Here's how the part is built. I have some questions about the finished solid (model axes, mm). Face numbers are marked on the shaded views. Give positions to 0.01 mm unless a question says otherwise; leave off trailing zeros. Order: outer loops, then holes, each group sorted by start corner. A loop starts at its lowest first (then second) coordinate and runs counter-clockwise, first axis right, second up.
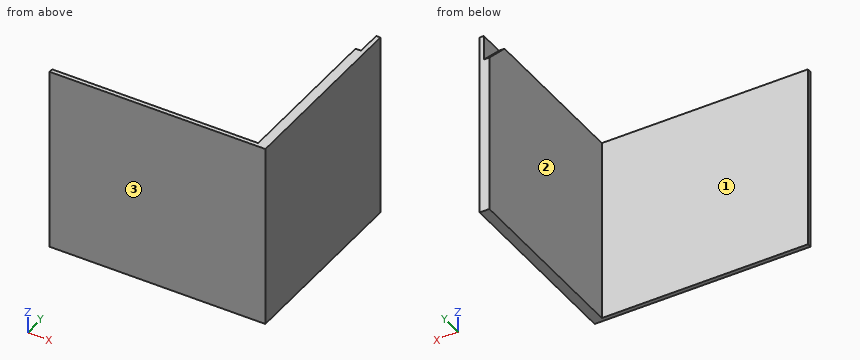
Autodesk Inventor part; units mm, degrees
ref_plane "YZ Plane" through (0, 0, 0) normal (1, 0, 0) x (0, 1, 0)
ref_plane "XZ Plane" through (0, 0, 0) normal (0, 1, 0) x (-1, 0, 0)
ref_plane "XY Plane" through (0, 0, 0) normal (0, 0, 1) x (1, 0, 0)
sketch "Sketch1" plane through (0, 0, 0) normal (0, 1, 0) x (-1, 0, 0)
  line L0 (110, -80) -> (-110, -80)
  line L1 (-110, -80) -> (-110, 80)
  line L2 (-110, 80) -> (110, 80)
  line L3 (110, 80) -> (110, -80)
  line L4 (320.2117, -53.5522) -> (168.036, -53.5522) construction
  line L5 (168.036, -53.5522) -> (168.036, 90.1689) construction
  line L6 (168.036, 90.1689) -> (320.2117, 90.1689) construction
  line L7 (320.2117, 90.1689) -> (320.2117, -53.5522) construction
  line L8 (124.3, -89.75) -> (-124.3, -89.75) construction
  line L9 (-124.3, -89.75) -> (-124.3, 89.75) construction
  line L10 (-124.3, 89.75) -> (124.3, 89.75) construction
  line L11 (124.3, 89.75) -> (124.3, -89.75) construction
  line L12 (124.3, -89.75) -> (-124.3, 89.75) construction
  line L13 (-124.3, -89.75) -> (124.3, 89.75) construction
  line L14 (-152.4, -107.95) -> (152.4, -107.95)
  line L15 (152.4, -107.95) -> (152.4, 107.95)
  line L16 (152.4, 107.95) -> (-152.4, 107.95)
  line L17 (-152.4, 107.95) -> (-152.4, -107.95)
  line L18 (-152.4, -107.95) -> (152.4, 107.95) construction
  line L19 (152.4, -107.95) -> (-152.4, 107.95) construction
  line L20 (177.8, 133.35) -> (177.8, -133.35)
  line L21 (177.8, -133.35) -> (-177.8, -133.35)
  line L22 (-177.8, -133.35) -> (-177.8, 133.35)
  line L23 (-177.8, 133.35) -> (177.8, 133.35)
  point P0 (0, 0)
  dimension "d11" = 220
  dimension "d12" = 160
  dimension "d15" = 248.6
  dimension "d16" = 179.5
  dimension "d18" = 304.8
  dimension "d19" = 215.9
  dimension "d22" = 25.4
extrude "Top" add sketch "Sketch1" along normal blind 25.4 contours L17 L16 L15 L14 | L20 L21 L22 L23
sketch "Sketch3" plane through (177.8, 0, 133.35) normal (1, 0, 0) x (0, 0, -1)
  line L0 (0, 0) -> (0, 25.4)
  line L1 (266.7, 0) -> (266.7, 25.4)
  line L2 (0, 0) -> (266.7, 0)
  line L3 (266.7, 0) -> (266.7, -266.7)
  line L4 (266.7, -266.7) -> (0, -266.7)
  line L5 (0, -266.7) -> (0, 0)
  point P0 (133.35, 0)
  dimension "d25" = 266.7
extrude "Right" add sketch "Sketch3" against normal blind 50.8
sketch "Sketch4" plane through (-177.8, 0, -133.35) normal (-1, 0, 0) x (0, 0, 1)
  line L0 (0, 0) -> (0, 25.4)
  line L1 (266.7, -266.7) -> (266.7, 0)
  line L2 (0, 0) -> (266.7, 0)
  line L3 (266.7, 0) -> (266.7, -266.7)
  line L4 (266.7, -266.7) -> (0, -266.7)
  line L5 (0, -266.7) -> (0, 0)
  point P0 (133.35, 0)
  dimension "d28" = 266.7
extrude "Left" add sketch "Sketch4" against normal blind 50.8
sketch "Sketch5" plane through (0, 0, 0) normal (1, 0, 0) x (0, 1, 0)
  line L0 (-266.7, -133.35) -> (25.4, -133.35)
  line L1 (-266.7, 133.35) -> (-266.7, -133.35)
  line L2 (0, -133.35) -> (-266.7, 133.35)
  line L3 (-266.7, 133.35) -> (-275.6803, 124.3697)
  line L4 (-275.6803, 124.3697) -> (-8.9803, -142.3303)
  line L5 (-8.9803, -142.3303) -> (0, -133.35)
  point P0 (0, 0)
  dimension "d31" = 12.7
extrude "Plexiglass Cut" cut sketch "Sketch5" along normal mid plane 304.8 contours L4 L1 L2 L0 | L0 L5 L4 | L4 L3 L1
sketch "Sketch6" plane through (-177.8, -266.7, -133.35) normal (0, -1, 0) x (1, 0, 0)
  line L0 (0, 0) -> (0, 266.7)
  line L1 (355.6, 0) -> (0, 0)
  line L2 (0, 266.7) -> (355.6, 266.7)
  line L3 (355.6, 266.7) -> (355.6, 0)
  line L4 (355.6, 0) -> (0, 0)
  line L5 (0, 0) -> (0, 266.7)
  point P0 (177.8, 133.35)
extrude "Bottom" add sketch "Sketch6" along normal blind 25.4
sketch "Sketch9" plane through (0, 25.4, 0) normal (0, 1, 0) x (1, 0, 0)
  line L0 (177.8, -133.35) -> (127, -133.35)
  line L1 (177.8, 133.35) -> (-177.8, 133.35)
  line L2 (177.8, -133.35) -> (-177.8, -133.35)
  line L3 (-177.8, -133.35) -> (-177.8, 133.35)
  line L4 (-177.8, 133.35) -> (177.8, 133.35)
  line L5 (177.8, 133.35) -> (177.8, -133.35)
  point P0 (0, 0)
extrude "Top Flattening" cut sketch "Sketch9" against normal blind 22.4
sketch "Sketch10" plane through (0, 3, 0) normal (0, 1, 0) x (1, 0, 0)
  line L0 (-177.8, -133.35) -> (-177.8, 133.35)
  line L1 (-155.4106, 133.35) -> (-177.8, 133.35)
  line L2 (-177.8, 133.35) -> (-177.8, -133.35)
  line L3 (-177.8, -133.35) -> (-155.4106, -133.35)
  line L4 (-155.4106, -133.35) -> (-155.4106, 133.35)
  line L5 (177.8, 133.35) -> (177.8, -133.35)
  line L6 (177.8, -133.35) -> (155.4106, -133.35)
  line L7 (155.4106, -133.35) -> (155.4106, 133.35)
  line L8 (155.4106, 133.35) -> (177.8, 133.35)
  line L9 (152.4, -115.3895) -> (152.4, 133.35)
  point P0 (0, 0)
  point P1 (-177.8, 0)
  dimension "d48" = 22.3894
  dimension "d49" = 22.3894
extrude "Outer Side Flattening" cut sketch "Sketch10" against normal through all
sketch "Sketch11" plane through (-177.8, -292.1, -133.35) normal (0, -1, 0) x (1, 0, 0)
  line L0 (22.3894, 0) -> (333.2106, 0)
  line L1 (333.2106, 0) -> (22.3894, 0)
  line L2 (22.3894, 0) -> (22.3894, 266.7)
  line L3 (22.3894, 266.7) -> (333.2106, 266.7)
  line L4 (333.2106, 266.7) -> (333.2106, 0)
  point P0 (177.8, 133.35)
extrude "Bottom Flattening" cut sketch "Sketch11" against normal blind 22.4
sketch "Sketch12" plane through (155.4106, 3, -133.35) normal (0, 0, -1) x (-1, 0, 0)
  line L0 (155.4106, -3) -> (155.4106, -269.7) construction
  line L1 (7.0106, -269.7) -> (7.0106, -3)
  line L2 (7.0106, -3) -> (303.8106, -3)
  line L3 (303.8106, -3) -> (303.8106, -269.7)
  line L4 (303.8106, -269.7) -> (7.0106, -269.7)
  line L5 (7.0106, -269.7) -> (303.8106, -3) construction
  line L6 (7.0106, -3) -> (303.8106, -269.7) construction
  point P0 (155.4106, -136.35)
  point P1 (155.4106, -3)
  dimension "d54" = 296.8
extrude "Inner Flattening" cut sketch "Sketch12" against normal through all
sketch "Sketch13" plane through (-155.4106, 3, 133.35) normal (0, 0, 1) x (1, 0, 0)
  line L0 (310.8211, -272.7) -> (310.8211, 0)
  line L1 (0, -272.7) -> (0, 0)
  line L2 (310.8211, -136.35) -> (0, -136.35)
  line L3 (0, -136.35) -> (0, 0)
  line L4 (0, 0) -> (310.8211, 0)
  line L5 (310.8211, 0) -> (310.8211, -136.35)
  point P0 (155.4106, -3)
  point P1 (310.8211, 0)
  point P2 (0, -136.35)
extrude "Top Cut" cut sketch "Sketch13" against normal through all
sketch "Sketch14" plane through (-155.4106, -133.35, 133.35) normal (0, 1, 0) x (1, 0, 0)
  line L0 (310.8211, 266.7) -> (0, 266.7)
  line L1 (155.4106, 133.35) -> (310.8211, 133.35)
  line L2 (310.8211, 133.35) -> (310.8211, 266.7)
  line L3 (310.8211, 266.7) -> (155.4106, 266.7)
  line L4 (155.4106, 266.7) -> (155.4106, 133.35)
  line L5 (0, 0) -> (310.8212, 0)
  line L6 (310.8211, 266.7) -> (0, 266.7)
  line L7 (0, 266.7) -> (0, 0)
  line L8 (0, 0) -> (310.8211, 0)
  line L9 (310.8211, 0) -> (310.8211, 266.7)
extrude "Quarter Cut" cut sketch "Sketch14" against normal through all contours L4 L1 L9 L5 L7 L0
properties part number "Apple iPad 2022 Hologram"
Q1. If we section it at A-A on z = -96: List the corners of the cut face in (x, y) for me, plus the area to 3 significant figures.
Filled sheet:
outline: (0, -269.7) - (155.41, -269.7) - (155.41, -133.35) - (148.4, -133.35) - (148.4, -266.7) - (0, -266.7) - close
area: 1,400 mm2
Q2. I need wall thicknesses on L1, parallel to X at y = -162, z = -77; L2, parallel to Y at x = 95, z = -104.5. Which ranges of each line are inside material? Lowest first, please.
Filled sheet:
L1: x = 148.4 to 155.41
L2: y = -269.7 to -266.7
Q3. If we section it at C-C on y = -229.5: List the corners of the cut face in (x, z) for me.
Filled sheet:
outline: (148.4, -133.35) - (155.41, -133.35) - (155.41, 0) - (148.4, 0) - close
Q4. Thinking about a two-plate mould opening in Y: for the marked faces 1, 2 and 3, which applies, released by +Y, released by -Y, zero draft, split by the parting line, or undercut?
Filled sheet:
face 1: released by +Y
face 2: zero draft
face 3: released by -Y
Q5. If we section it at B-B on x = 17: List the corners of the cut face in (y, z) for me.
Filled sheet:
outline: (-269.7, -133.35) - (-266.7, -133.35) - (-266.7, 0) - (-269.7, 0) - close
Q6. I'm going to push flat-ended pins straight in: P1, Ø3, axis at x = 60, z = -36, coming from the +Y side; P2, Ø2, axis at y = -186, z = -79, coming from the -X side. Where does each tip first touch, or does it pass through?
Filled sheet:
P1: stops at y = -266.7
P2: stops at x = 148.4
